Geometry: final body of the model. Coordinates: model frame, mm. Coordinates: 2 decimals unless noted, no trailing zeros. Order: outer loops, then holes, each group sorted by start corner. A loop starts at its lowest first (then second) coordinate and runs counter-clockwise, first axis right, second up. Notation, with made-up numbers: M 68.25,-24 L 124.25,-24 A16 ccw 124.25,-16 Z; hole C 53,22 d2. An arc over 180 degrees is marked long. Write item = value, one per line.
from build123d import *

# Parameters (mm, degrees)
SKETCH1_W           = 465
SKETCH1_H           = 90
SKETCH1_R           = 2.55
BOSS_EXTRUDE1_DEPTH = 2.2479
SKETCH2_R           = 4.7625
CUT_EXTRUDE1_DEPTH  = 4.4958


with BuildPart() as part:
    # Sketch1 → Boss-Extrude1 (new body, symmetric)
    with BuildSketch(Plane.XY):
        Rectangle(SKETCH1_W, SKETCH1_H)
        with Locations((-222.5, 35)):
            Circle(SKETCH1_R, mode=Mode.SUBTRACT)
        with Locations((-222.5, -35)):
            Circle(SKETCH1_R, mode=Mode.SUBTRACT)
        with Locations((0, 35)):
            Circle(SKETCH1_R, mode=Mode.SUBTRACT)
        with Locations((-114.975, 35)):
            Circle(SKETCH1_R, mode=Mode.SUBTRACT)
        with Locations((222.5, -35)):
            Circle(SKETCH1_R, mode=Mode.SUBTRACT)
        with Locations((222.5, 35)):
            Circle(SKETCH1_R, mode=Mode.SUBTRACT)
        with Locations((114.975, 35)):
            Circle(SKETCH1_R, mode=Mode.SUBTRACT)
    extrude(amount=BOSS_EXTRUDE1_DEPTH, both=True)

    # Sketch2 → Cut-Extrude1 (cut)
    with BuildSketch(Plane.XY.offset(2.2479)):
        with Locations((0, 15)):
            Circle(SKETCH2_R)
        with Locations((15, 15)):
            Circle(SKETCH2_R)
        with Locations((30, 15)):
            Circle(SKETCH2_R)
        with Locations((45, 15)):
            Circle(SKETCH2_R)
        with Locations((60, 15)):
            Circle(SKETCH2_R)
        with Locations((75, 15)):
            Circle(SKETCH2_R)
        with Locations((15, 0)):
            Circle(SKETCH2_R)
        with Locations((30, 0)):
            Circle(SKETCH2_R)
        with Locations((45, 0)):
            Circle(SKETCH2_R)
        with Locations((60, 0)):
            Circle(SKETCH2_R)
        with Locations((75, 0)):
            Circle(SKETCH2_R)
        with Locations((15, -15)):
            Circle(SKETCH2_R)
        with Locations((30, -15)):
            Circle(SKETCH2_R)
        with Locations((45, -15)):
            Circle(SKETCH2_R)
        with Locations((60, -15)):
            Circle(SKETCH2_R)
        with Locations((75, -15)):
            Circle(SKETCH2_R)
        with Locations((15, -30)):
            Circle(SKETCH2_R)
        with Locations((30, -30)):
            Circle(SKETCH2_R)
        with Locations((45, -30)):
            Circle(SKETCH2_R)
        with Locations((60, -30)):
            Circle(SKETCH2_R)
        with Locations((75, -30)):
            Circle(SKETCH2_R)
        Circle(SKETCH2_R)
        with Locations((0, -15)):
            Circle(SKETCH2_R)
        with Locations((0, -30)):
            Circle(SKETCH2_R)
        with Locations((-75, -30)):
            Circle(SKETCH2_R)
        with Locations((-60, -30)):
            Circle(SKETCH2_R)
        with Locations((-45, -30)):
            Circle(SKETCH2_R)
        with Locations((-30, -30)):
            Circle(SKETCH2_R)
        with Locations((-15, -30)):
            Circle(SKETCH2_R)
        with Locations((-75, -15)):
            Circle(SKETCH2_R)
        with Locations((-60, -15)):
            Circle(SKETCH2_R)
        with Locations((-45, -15)):
            Circle(SKETCH2_R)
        with Locations((-30, -15)):
            Circle(SKETCH2_R)
        with Locations((-15, -15)):
            Circle(SKETCH2_R)
        with Locations((-75, 0)):
            Circle(SKETCH2_R)
        with Locations((-60, 0)):
            Circle(SKETCH2_R)
        with Locations((-45, 0)):
            Circle(SKETCH2_R)
        with Locations((-30, 0)):
            Circle(SKETCH2_R)
        with Locations((-15, 0)):
            Circle(SKETCH2_R)
        with Locations((-75, 15)):
            Circle(SKETCH2_R)
        with Locations((-60, 15)):
            Circle(SKETCH2_R)
        with Locations((-45, 15)):
            Circle(SKETCH2_R)
        with Locations((-30, 15)):
            Circle(SKETCH2_R)
        with Locations((-15, 15)):
            Circle(SKETCH2_R)
    extrude(amount=-CUT_EXTRUDE1_DEPTH, mode=Mode.SUBTRACT)


solid = part.part
1) Section A-A, the plane x = 30. Return loops of the section in (y, z).
Numbers:
outline = M -45,-2.25 L -34.76,-2.25 L -34.76,2.25 L -45,2.25 Z; M -25.24,-2.25 L -19.76,-2.25 L -19.76,2.25 L -25.24,2.25 Z; M -10.24,-2.25 L -4.76,-2.25 L -4.76,2.25 L -10.24,2.25 Z; M 4.76,-2.25 L 10.24,-2.25 L 10.24,2.25 L 4.76,2.25 Z; M 19.76,-2.25 L 45,-2.25 L 45,2.25 L 19.76,2.25 Z
2) Pin query (flat end, axial travel): pin 1 (5.5 mm diameter, centred on x = 30, y = 15, fed in from +Z); pin 2 (12.5 mm diameter, centred on x = -75, y = 0, fed in from +Z). Return the tip coordinate at first contact, or that it passes through.
Numbers:
pin_1 = through
pin_2 = 2.25
3) Line query: L1, parallel to Y at x = 29.5, z = 0.65; L2, parallel to Y at x = -222.5, z = -0.4; L3, parallel to Y at x = -45, z = 0.75. Output: solid intervals per line, ascending.
Numbers:
L1 = -45 to -34.74, -25.26 to -19.74, -10.26 to -4.74, 4.74 to 10.26, 19.74 to 45
L2 = -45 to -37.55, -32.45 to 32.45, 37.55 to 45
L3 = -45 to -34.76, -25.24 to -19.76, -10.24 to -4.76, 4.76 to 10.24, 19.76 to 45
4) Section B-B, the plane z = -0.2. Give the number of separate pieces and of enclosed holes in the cut face, and give its area (3 significant figures).
Numbers:
separate_pieces = 1
enclosed_holes = 51
area = 38,600 mm²
